from build123d import *

# Parameters (mm, degrees)
SKETCH1_W               = 62.4208
SKETCH1_H               = 60
SKETCH1_R               = 13.5
BOSS_EXTRUDE1_DEPTH     = 1
BOSS_EXTRUDE2_START     = -1
SKETCH2_W               = 53.9308
SKETCH2_H               = 4.6
BOSS_EXTRUDE2_DEPTH     = 7
BOSS_EXTRUDE3_DEPTH     = 14
BOSS_EXTRUDE4_DEPTH     = 1
CUT_EXTRUDE1_REACH      = 103.509
CUT_EXTRUDE1_END_RADIUS = 57.5


with BuildPart() as part:
    # Sketch1 → Boss-Extrude1 (new body)
    with BuildSketch(Plane.XY):
        with Locations((6.283906244, 0.094262462)):
            Rectangle(SKETCH1_W, SKETCH1_H)
        with Locations((15.494306244, 0.094262462)):
            Circle(SKETCH1_R, mode=Mode.SUBTRACT)
    extrude(amount=BOSS_EXTRUDE1_DEPTH)

    # Sketch2 → Boss-Extrude2 (add)
    with BuildSketch(Plane.XY.offset(1).offset(BOSS_EXTRUDE2_START)):
        with Locations((2.038906244, -27.605737538)):
            Rectangle(SKETCH2_W, SKETCH2_H)
        with Locations((2.038906244, 27.794262462)):
            Rectangle(SKETCH2_W, SKETCH2_H)
    extrude(amount=-BOSS_EXTRUDE2_DEPTH)



with BuildPart() as body_2:
    # Sketch3 → Boss-Extrude3 (new body)
    with BuildSketch(Plane.XY.offset(1)):
        with BuildLine():
            ThreePointArc((-33.559235932, 30.094262462), (-24.010484349, 41.87489817), (-11.714027053, 50.749534638))
            Line((-11.714027053, 50.749534638), (-16.003239131, 58.735000077))
            ThreePointArc((-16.003239131, 58.735000077), (-32.167096843, 46.561693298), (-43.926493756, 30.094262462))
            Line((-43.926493756, 30.094262462), (-33.559235932, 30.094262462))
        make_face()
        with BuildLine():
            Line((-43.926493756, -29.905737538), (-33.559235932, -29.905737538))
            ThreePointArc((-33.559235932, -29.905737538), (-42.005693756, 0.094262462), (-33.559235932, 30.094262462))
            Line((-33.559235932, 30.094262462), (-43.926493756, 30.094262462))
            Line((-43.926493756, 30.094262462), (-43.926493756, -29.905737538))
        make_face()
        with BuildLine():
            Line((-16.003239131, -58.546475153), (-11.714027053, -50.561009713))
            ThreePointArc((-11.714027053, -50.561009713), (-24.010484349, -41.686373246), (-33.559235932, -29.905737538))
            Line((-33.559235932, -29.905737538), (-43.926493756, -29.905737538))
            ThreePointArc((-43.926493756, -29.905737538), (-32.167096843, -46.373168373), (-16.003239131, -58.546475153))
        make_face()
    extrude(amount=BOSS_EXTRUDE3_DEPTH)


with BuildPart() as part_1:
    add(part.part)

    add(body_2.part)  # Boss-Extrude4 merges body 2
    # Sketch4 → Boss-Extrude4 (add)
    with BuildSketch(Plane.XY.offset(1)):
        with BuildLine():
            Line((37.494306244, -42.119641485), (37.494306244, -29.905737538))
            Line((37.494306244, -29.905737538), (-24.926493756, -29.905737538))
            Line((-24.926493756, -29.905737538), (-24.926493756, 30.094262462))
            Line((-24.926493756, 30.094262462), (37.494306244, 30.094262462))
            Line((37.494306244, 30.094262462), (37.494306244, 42.30816641))
            ThreePointArc((37.494306244, 42.30816641), (15.197309329, 47.696000659), (-7.030722747, 42.030365708))
            Line((-7.030722747, 42.030365708), (-16.003239131, 58.735000077))
            ThreePointArc((-16.003239131, 58.735000077), (-32.167096843, 46.561693298), (-43.926493756, 30.094262462))
            Line((-43.926493756, 30.094262462), (-43.926493756, -29.905737538))
            ThreePointArc((-43.926493756, -29.905737538), (-32.167096843, -46.373168373), (-16.003239131, -58.546475153))
            Line((-16.003239131, -58.546475153), (-7.030722747, -41.841840784))
            ThreePointArc((-7.030722747, -41.841840784), (15.197309329, -47.507475734), (37.494306244, -42.119641485))
        make_face()
    extrude(amount=-BOSS_EXTRUDE4_DEPTH)

    # Cut-Extrude1: up to this cylinder (the profile starts outside it)
    cut_extrude1_end = Plane(origin=(15.494306244, 0.094262462, 7.5), z_dir=(0, 0, -1)) * Cylinder(CUT_EXTRUDE1_END_RADIUS, 323.018, mode=Mode.PRIVATE)
    # Sketch5 → Cut-Extrude1 (cut, up to the surface)
    with BuildSketch(Plane.ZY.offset(43.926493756), mode=Mode.PRIVATE) as cut_extrude1_sk1:
        with BuildLine():
            Line((4, 2.25), (11, 2.25))
            ThreePointArc((11, 2.25), (13.25, 0), (11, -2.25))
            Line((11, -2.25), (4, -2.25))
            ThreePointArc((4, -2.25), (1.75, 0), (4, 2.25))
        make_face()
    cut_extrude1_tool1 = extrude(cut_extrude1_sk1.sketch, amount=-CUT_EXTRUDE1_REACH, mode=Mode.PRIVATE) - cut_extrude1_end
    add(cut_extrude1_tool1.solids().sort_by_distance((-43.926494, 0, 7.5))[0], mode=Mode.SUBTRACT)


solid = part_1.part
The listing builds one solid part. Answer for the finished solid, in the listing's coordinates (mm). A direction names the side the tool comes from. Coordinates: 2 decimals unless noted, no trailing zeros. Write each loop counter-clockwise with the first axis right and the second up, starting at its lowest first coordinate (ties: lowest second). Pieces come first, ordered by that corner, then holes. Notation, with made-up numbers: M -5,23 L 19,23 A32 cw 19,52 Z; hole C -9,33.25 d1. An arc over 180 degrees is marked long. Put each result on its own line as item: value. Start each with the question number.
1. A cutting plane is placed at B-B on y = 44.5. Write down the section's boundary in (x, z).
2. Which of the six approach directions +Z, -Z, +X, -X, +Y, -Y give full straight-line access (tool end or side, diameter ignored) to faces 1 (the flat face through (2, 25.494, -3)), 2 (the flat face through (2, -29.906, -3)), 3 (the cylindrical face through (-42.96, 0.05, 13.25)), 4 (the flat face through (-3, 1, 1))?
3. Consider line 1 (Y direction, x = -17, z = -3.25); line 2 (Z direction, x = 14, y = -47); line 3 (Z direction, x = -33, y = 35). Determine where each line is inside the solid, lowest interval first. Write a range as from..to.
4. Flat-ended cylindrical pins translate along their axes: P1, Ø7.5, axis at x = -9.5, z = -4, coming from the +Y side; P2, Ø24.5, axis at x = -19, y = -12, coming from the -Z side; P3, Ø8, axis at x = -2, y = 20, coming from the +Z side; P4, Ø16, axis at x = 15.49, y = 0.09, coming from the -Z side. Find the tip coordinate at first contact, or state that the pin passes through.
5. A cutting plane is placed at C-C on x = -28. Write down the section's boundary in (y, z) (3 decimals), then the cut area to 3 significant figures.
6. A cutting plane is placed at D-D on y = 32. Write down the section's boundary in (x, z), then the cut area to 3 significant figures.
7. For a pull along Y with two mould halves and no side action, classify faces 5 (the cylindrical face through (-32.365, -46.169, 7.605)), 6 (the cylindrical face through (-31.968, 46.765, 7.605)), 7 (the flat face through (2, -25.306, -3)), 8 (the flat face through (-24.926, 28, -3)) as pulls with the +Y half, pulls with the -Y half, needs draft (parallel to the pull), parting line crosses it, or undercut.
Resolved:
1. outline: M -34.09,0 L -8.36,0 L -8.36,1 L -21.03,1 L -21.03,15 L -34.09,15 Z; M -1.66,0 L 32.64,0 L 32.64,1 L -1.66,1 Z
2. face 1: -Z, +X, -X
2. face 2: -Z, +X, -X, -Y
2. face 3: +X, -X
2. face 4: +Z, +X
3. line 1: y = -29.91..-25.31, 25.49..30.09
3. line 2: z = 0..1
3. line 3: z = 0..15
4. P1: stops at y = 30.09
4. P2: stops at z = 0
4. P3: stops at z = 1
4. P4: passes through
5. outline: M -50.295,0 L 50.484,0 L 50.484,15 L 37.704,15 L 37.704,1 L -37.516,1 L -37.516,15 L -50.295,15 Z
5. area: 459 mm2
6. outline: M -42.93,0 L 37.49,0 L 37.49,1 L -32.34,1 L -32.34,15 L -42.93,15 Z
6. area: 229 mm2
7. face 5: pulls with the -Y half
7. face 6: pulls with the +Y half
7. face 7: undercut
7. face 8: needs draft
